For this review, use the dimensioned drawing (mm, ordinates from the lowest corner) and the shaded views. A direction names the side the tool comes from. Give positions to 0.01 mm unless a question says otherwise; leave off trailing zeros. Write each loop counter-clockwise with the first axis right and the second up, starting at its lowest first coordinate (ties: lowest second). Pieces come first, ordered by that corner, then holes. Notation, with made-up numbers: (-23, 6.25) -> (2, 6.25) arc R30 ccw to (2, 42.25) -> close; hole circle Ø8 at (43, -40). An arc over 180 degrees is marked (long way). Write each question's results on one line, items separated by ' | '. Start each with the question number.
(1) Mouldability with a two-part tool opening along Y and no side actions: class the marked faces 3, 4 and 5 as released by +Y, released by -Y, zero draft, split by the parting line, or undercut.
(2) For the marked faces 1 and 2, list the 3-axis set-ups (+Z, -Z, +X, -X, +Y, -Y) from which the entire face can be reached by the end or side of a thin tool; tool diameter is ignored.
(3) Take a section at A-A (y = 4.75). State the section outline as (x, z) points.
(4) Take a section at B-B (x = 3.25). State the section outline as (y, z) points, plus the area to 3 significant figures.
(5) Take a section at D-D (x = 6). State the section outline as (y, z) points.
(6) Take a section at C-C (z = 6). State the section outline as (x, y) points, plus the area to 3 significant figures.
(7) Clearance check with flat-ended pins moving along their axes: pin 1 (2 mm diameter, centred on x = 7.5, z = 7.5, fed in from -Y); pin 2 (1.2 mm diameter, centred on y = 3, z = 9, fed in from -X). State where each tip first meets the part, or that it passes through.
(8) To check wall thickness, follow probe 1 along Y at (x, z) = (3.25, 14); probe 2 along X at (y, z) = (4.5, 22.25); probe 3 along Y at (x, z) = (14, 4.25). State the ranges of each line that lie inside material, in increasing order.
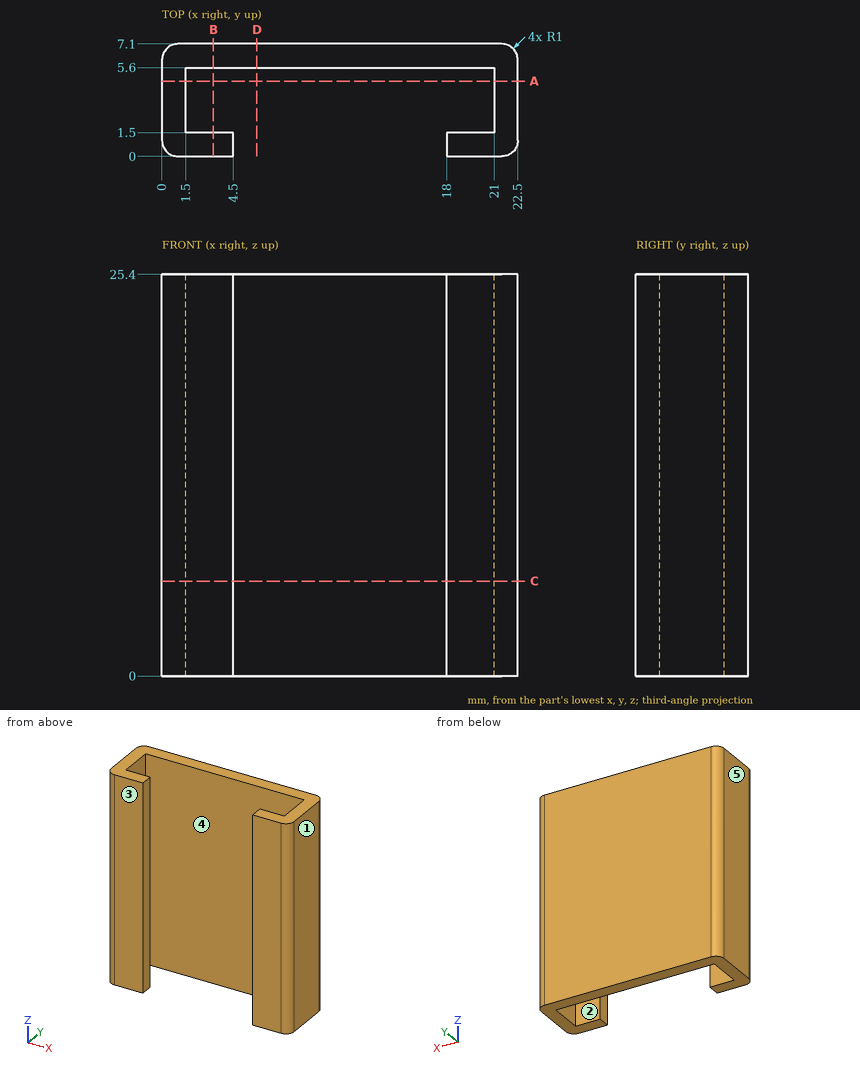
Report:
1) face 3: released by -Y | face 4: undercut | face 5: zero draft
2) face 1: +Z, -Z, +X, +Y, -Y | face 2: +Z, -Z
3) outline: (0, 0) -> (1.5, 0) -> (1.5, 25.4) -> (0, 25.4) -> close; (21, 0) -> (22.5, 0) -> (22.5, 25.4) -> (21, 25.4) -> close
4) outline: (0, 0) -> (1.5, 0) -> (1.5, 25.4) -> (0, 25.4) -> close; (5.6, 0) -> (7.1, 0) -> (7.1, 25.4) -> (5.6, 25.4) -> close | area: 76.2 mm2
5) outline: (5.6, 0) -> (7.1, 0) -> (7.1, 25.4) -> (5.6, 25.4) -> close
6) outline: (0, 1) arc R1 ccw to (1, 0) -> (4.5, 0) -> (4.5, 1.5) -> (1.5, 1.5) -> (1.5, 5.6) -> (21, 5.6) -> (21, 1.5) -> (18, 1.5) -> (18, 0) -> (21.5, 0) arc R1 ccw to (22.5, 1) -> (22.5, 6.1) arc R1 ccw to (21.5, 7.1) -> (1, 7.1) arc R1 ccw to (0, 6.1) -> close | area: 58.7 mm2
7) pin 1: y = 5.6 | pin 2: x = 0
8) probe 1: 0 to 1.5, 5.6 to 7.1 | probe 2: 0 to 1.5, 21 to 22.5 | probe 3: 5.6 to 7.1
